```python
from build123d import *

# Parameters (mm, degrees)
BOSS_EXTRUDE1_DEPTH      = 2
CUT_EXTRUDE2_DEPTH       = 2
FILL_START               = 36.116581205
FILL_PATTERN1_DEPTH      = 2
BOSS_EXTRUDE2_DEPTH      = 2
BOSS_EXTRUDE2_DEPTH_BACK = 2


# Read off the part's stored shape, not the designer's step: Fill Pattern1
with BuildPart() as part:
    # Sketch1 → Boss-Extrude1 (new body)
    with BuildSketch(Plane(origin=(33.669790065, -11.316558939, 6.533618345), x_dir=(0.3075963595688898, 0.9496429323114018, 0.059689033255435724), z_dir=(0.9322529691900319, -0.3133341684384297, 0.1809035663699512))):
        with BuildLine():
            Line((-57.568945453, 121.68686406), (-100.902387075, 51.715943852))
            Line((-100.902387075, 51.715943852), (-100.902387075, 32.254389388))
            add(Edge.make_bspline(
                [(-100.902387075, 32.254389388), (-100.442473357, 31.458808563), (-99.383581078, 29.928136313), (-97.483264926, 27.996228976), (-95.226180551, 26.317886768), (-92.562665334, 24.828690878), (-89.619940932, 23.519356376), (-86.433701886, 22.304158353), (-83.615975501, 21.289615886), (-81.305064927, 20.428782251), (-80.113678401, 19.962997336), (-79.526238835, 19.725091457)],
                knots=[0.001143674, 0.001143674, 0.001143674, 0.001143674, 0.119233579, 0.237323485, 0.35541339, 0.473503295, 0.5915932, 0.709683105, 0.82777301, 0.886817963, 0.945862915, 0.945862915, 0.945862915, 0.945862915], degree=3))
            Line((-79.526238835, 19.725091457), (-17.875333173, 119.273395013))
            Line((-17.875333173, 119.273395013), (-57.568945453, 121.68686406))
        make_face()
    extrude(amount=BOSS_EXTRUDE1_DEPTH)

    # Sketch2 → Cut-Extrude2 (cut)
    with BuildSketch(Plane(origin=(35.534296004, -11.943227276, 6.895425478), x_dir=(0.30759635956877757, 0.9496429323114396, 0.05968903325541397), z_dir=(0.9322529691900542, -0.3133341684383154, 0.18090356637003419))):
        Polygon((-60.882260573, 113.944557721), (-59.845221607, 108.206275442), (-54.357203896, 106.235236392), (-49.906225151, 110.002479621), (-50.943264117, 115.7407619), (-56.431281828, 117.71180095), align=None)
    extrude(amount=-CUT_EXTRUDE2_DEPTH, mode=Mode.SUBTRACT)

    # Fill Pattern1 outline → Fill Pattern1 (cut)
    with BuildSketch(Plane(origin=(0, 0, 0), x_dir=(0.3075963595751989, 0.9496429323114397, 0.05968903322232153), z_dir=(0.9322529691900542, -0.31333416843831513, 0.18090356637003466)).offset(FILL_START)):
        Polygon((-82.988049322, 35.354420584), (-87.439028067, 31.587177355), (-86.4019891, 25.848895075), (-80.913971389, 23.877856025), (-76.462992645, 27.645099254), (-77.500031611, 33.383381534), align=None)
        Polygon((-38.760899761, 106.768419503), (-43.211878505, 103.001176274), (-42.174839539, 97.262893995), (-36.686821828, 95.291854945), (-32.235843083, 99.059098174), (-33.27288205, 104.797380453), align=None)
        Polygon((-50.755172908, 107.139110303), (-55.206151653, 103.371867074), (-54.169112686, 97.633584795), (-48.681094975, 95.662545745), (-44.230116231, 99.429788974), (-45.267155197, 105.168071253), align=None)
        Polygon((-45.079063984, 96.566419658), (-49.530042728, 92.799176429), (-48.493003762, 87.060894149), (-43.004986051, 85.089855099), (-38.554007306, 88.857098328), (-39.591046273, 94.595380608), align=None)
        Polygon((-62.749446055, 107.509801103), (-67.2004248, 103.742557873), (-66.163385834, 98.004275594), (-60.675368123, 96.033236544), (-56.224389378, 99.800479773), (-57.261428344, 105.538762052), align=None)
        Polygon((-44.437008685, 117.341110149), (-48.88798743, 113.573866919), (-47.850948463, 107.83558464), (-42.362930752, 105.86454559), (-37.911952008, 109.631788819), (-38.948990974, 115.370071098), align=None)
        Polygon((-32.442735538, 116.970419349), (-36.893714282, 113.20317612), (-35.856675316, 107.464893841), (-30.368657605, 105.493854791), (-25.91767886, 109.26109802), (-26.954717827, 114.999380299), align=None)
        Polygon((-88.022102947, 66.70180172), (-92.473081692, 62.934558491), (-91.436042726, 57.196276212), (-85.948025015, 55.225237161), (-81.49704627, 58.992480391), (-82.534085236, 64.73076267), align=None)
        Polygon((-70.351720876, 55.758420275), (-74.802699621, 51.991177046), (-73.765660654, 46.252894767), (-68.277642943, 44.281855717), (-63.826664199, 48.049098946), (-64.863703165, 53.787381225), align=None)
        Polygon((-81.703938724, 76.903801566), (-86.154917469, 73.136558336), (-85.117878503, 67.398276057), (-79.629860792, 65.427237007), (-75.178882047, 69.194480236), (-76.215921013, 74.932762515), align=None)
        Polygon((-76.0278298, 66.33111092), (-80.478808545, 62.563867691), (-79.441769579, 56.825585412), (-73.953751868, 54.854546362), (-69.502773123, 58.621789591), (-70.539812089, 64.36007187), align=None)
        Polygon((-94.34026717, 56.499801874), (-98.791245915, 52.732558645), (-97.754206949, 46.994276366), (-92.266189238, 45.023237316), (-87.815210493, 48.790480545), (-88.852249459, 54.528762824), align=None)
        Polygon((-88.664158246, 45.927111229), (-93.115136991, 42.159868), (-92.078098025, 36.421585721), (-86.590080314, 34.450546671), (-82.139101569, 38.2177899), (-83.176140535, 43.956072179), align=None)
        Polygon((-82.345994023, 56.129111075), (-86.796972768, 52.361867846), (-85.759933802, 46.623585566), (-80.271916091, 44.652546516), (-75.820937346, 48.419789745), (-76.857976312, 54.158072025), align=None)
        Polygon((-76.669885099, 45.556420429), (-81.120863844, 41.7891772), (-80.083824877, 36.050894921), (-74.595807166, 34.079855871), (-70.144828422, 37.8470991), (-71.181867388, 43.585381379), align=None)
        Polygon((-69.067610278, 97.307801257), (-73.518589023, 93.540558028), (-72.481550057, 87.802275749), (-66.993532346, 85.831236698), (-62.542553601, 89.598479928), (-63.579592567, 95.336762207), align=None)
        Polygon((-63.391501354, 86.735110612), (-67.842480099, 82.967867383), (-66.805441132, 77.229585103), (-61.317423421, 75.258546053), (-56.866444677, 79.025789282), (-57.903483643, 84.764071561), align=None)
        Polygon((-57.073337131, 96.937110457), (-61.524315876, 93.169867228), (-60.487276909, 87.431584949), (-54.999259198, 85.460545899), (-50.548280454, 89.227789128), (-51.58531942, 94.966071407), align=None)
        Polygon((-51.397228207, 86.364419812), (-55.848206951, 82.597176583), (-54.811167985, 76.858894304), (-49.323150274, 74.887855254), (-44.872171529, 78.655098483), (-45.909210496, 84.393380762), align=None)
        Polygon((-69.709665577, 76.533110766), (-74.160644322, 72.765867537), (-73.123605356, 67.027585258), (-67.635587645, 65.056546208), (-63.1846089, 68.823789437), (-64.221647866, 74.562071716), align=None)
        Polygon((-64.033556653, 65.960420121), (-68.484535398, 62.193176892), (-67.447496431, 56.454894612), (-61.95947872, 54.483855562), (-57.508499976, 58.251098791), (-58.545538942, 63.989381071), align=None)
        Polygon((-75.385774501, 87.105801411), (-79.836753246, 83.338558182), (-78.79971428, 77.600275903), (-73.311696569, 75.629236853), (-68.860717824, 79.396480082), (-69.89775679, 85.134762361), align=None)
        Polygon((-57.71539243, 76.162419966), (-62.166371175, 72.395176737), (-61.129332208, 66.656894458), (-55.641314497, 64.685855408), (-51.190335753, 68.453098637), (-52.227374719, 74.191380916), align=None)
    extrude(amount=FILL_PATTERN1_DEPTH, mode=Mode.SUBTRACT)

    # Sketch3 → Boss-Extrude2 (add, two sides: drawn at the far end of the back side and taken through both)
    with BuildSketch(Plane(origin=(35.534296004, -11.943227276, 6.895425478), x_dir=(0.3075963595751957, 0.9496429323114406, 0.05968903322232247), z_dir=(0.9322529691900543, -0.31333416843831224, 0.1809035663700394)).offset(-BOSS_EXTRUDE2_DEPTH_BACK)):
        Polygon((-68.737584877, 103.652755792), (-29.043972597, 101.239286747), (-49.359262726, 68.435994613), (-89.052875005, 70.849463659), align=None)
    extrude(amount=BOSS_EXTRUDE2_DEPTH + BOSS_EXTRUDE2_DEPTH_BACK)


solid = part.part
```
Work out the finished part from the listing and answer in its coordinate system (mm). A direction names the side the tool comes from. Round coordinates to 2 decimals unless told otherwise and drop trailing zeros. Loops run counter-clockwise (first coordinate to the right, second up) from the corner with the lowest first, then second, coordinate; pieces in that order, holes last. Notation, with made-up numbers: (24, 53.25) -> (51, 53.25) arc R23 cw to (51, 88.25) -> close; hole circle Ø6 at (58.25, 85). An arc over 180 degrees is marked (long way). Write each question's results on one line, items separated by ' | '. Start each with the question number.
1. Section A-A (z = 102.5) is taken. Determine the outline of the cut face in (x, y), plus the area to 3 significant figures.
2. Find the intervals of material crossed by probe 1 along Y at (x, z) = (-1, 59); probe 2 along X at (y, z) = (-73.5, 109.5); probe 3 along X at (y, z) = (-101, 28), in increasing order. Write a range as from..to.
3. A tool of negligible diameter and unlimited length cuts with its end or side. For faces 1 (the face through (1.71, -91.77, 37.32)), 2 (the face through (-1.75, -97.91, 44.55)), from which of +Z, -Z, +X, -X, +Y, -Y can it reach the whole face along a straight path? Write none if from no direction.
4. For a pull along Y with two mould halves and no side action, classify faces 3 (the face through (0.16, -70.82, 76.15)), 4 (the face through (-2.803, -65.776, 105.614)), 5 (the face through (1.347, -84.114, 52.466)) as +Y half, -Y half, draft (parallel to the pull), parting line (faces both ways), or undercut.
5. Given pin 1 Ø2 at (y, z) = (-59, 92.5) entering from -X; pin 2 Ø2 at (x, z) = (7, 66) entering from +Y; pin 3 Ø5 at (y, z) = (-89, 60) entering from -X, each flat-ended and moving along its own axis, determine where each tip first touches the part or whether it passes through.
Evaluation:
1) outline: (-7.22, -77.57) -> (-3.49, -79.24) -> (9.18, -41.54) -> (5.45, -39.87) -> close | area: 162 mm2
2) probe 1: y = -90.3..-87.28 | probe 2: x = -7.21..-5.07 | probe 3: x = -0.64..1.51
3) face 1: -X | face 2: +X
4) face 3: +Y half | face 4: undercut | face 5: -Y half
5) pin 1: stops at x = 0.57 | pin 2: stops at y = -60.91 | pin 3: stops at x = -3.37
